Build history of the part. All positions in model axes, mm. Face numbers are marked on the shaded views. A direction names the side the tool comes from. Give positions to 0.01 mm unless a question says otherwise; leave off trailing zeros. Order: outer loops, then holes, each group sorted by start corner. A loop starts at its lowest first (then second) coordinate and runs counter-clockwise, first axis right, second up. Notation, with made-up numbers: M 54.5,51 L 77.5,51 A10 ccw 77.5,56 Z; hole C 29.25,-19 d8. An arc over 180 degrees is marked long. One line per item, written item: value.
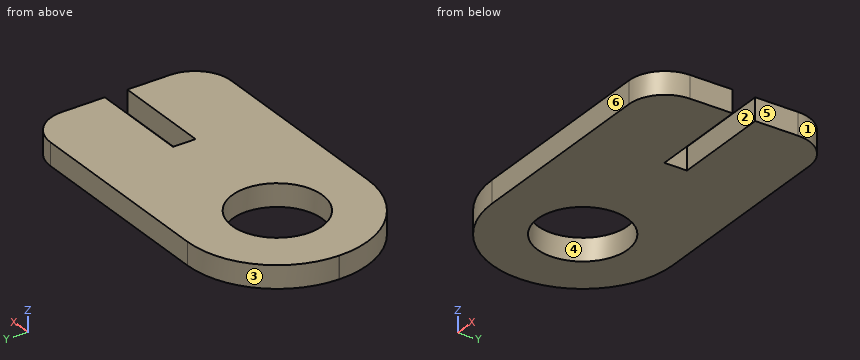
from build123d import *

# Parameters (mm, degrees)
SKETCH1_R           = 3.175
BOSS_EXTRUDE1_DEPTH = 1.5875


with BuildPart() as part:
    # Sketch1 → Boss-Extrude1 (new body)
    with BuildSketch(Plane.XY):
        with BuildLine():
            Line((-0.0254, 6.35), (13.97, 6.35))
            ThreePointArc((13.97, 6.35), (15.766051224, 5.606051224), (16.51, 3.81))
            Line((16.51, 3.81), (16.51, 0.79375))
            Line((16.51, 0.79375), (9.525, 0.79375))
            Line((9.525, 0.79375), (9.525, -0.79375))
            Line((9.525, -0.79375), (16.51, -0.79375))
            Line((16.51, -0.79375), (16.51, -3.81))
            ThreePointArc((16.51, -3.81), (15.766051224, -5.606051224), (13.97, -6.35))
            Line((13.97, -6.35), (-0.0254, -6.35))
            ThreePointArc((-0.0254, -6.35), (-4.497567548, -4.497567548), (-6.35, -0.0254))
            Line((-6.35, -0.0254), (-6.35, 0.0254))
            ThreePointArc((-6.35, 0.0254), (-4.497567548, 4.497567548), (-0.0254, 6.35))
        make_face()
        Circle(SKETCH1_R, mode=Mode.SUBTRACT)
    extrude(amount=BOSS_EXTRUDE1_DEPTH)


solid = part.part
1) Saw through at C-C, the plane x = 2.5. Write the cut outline in (y, z).
Check values:
outline: M -6.35,0 L -1.96,0 L -1.96,1.59 L -6.35,1.59 Z; M 1.96,0 L 6.35,0 L 6.35,1.59 L 1.96,1.59 Z
2) Saw through at A-A, the plane x = 11. Write the cut outline in (y, z), then the cut area to 3 significant figures.
Check values:
outline: M -6.35,0 L -0.79,0 L -0.79,1.59 L -6.35,1.59 Z; M 0.79,0 L 6.35,0 L 6.35,1.59 L 0.79,1.59 Z
area: 17.6 mm^2
3) Mould opens along X. For the marked faces 3, 4, 5 and 6 say: released by +X, released by -X, zero draft, split by the parting line, or undercut.
Check values:
face 3: released by -X
face 4: undercut
face 5: released by +X
face 6: zero draft
4) Tool access for the marked faces 1 and 2: list every direction of +Z, -Z, +X, -X, +Y, -Y with a clear straight run to the whole face (end or side of a thin tool).
Check values:
face 1: +Z, -Z, +X, +Y
face 2: +Z, -Z, +X
5) Saw through at B-B, the plane z = 1.05. Write the cut outline in (x, y) (3 decimals), then the cut area to 3 significant figures.
Check values:
outline: M -6.35,-0.025 A6.325 ccw -0.025,-6.35 L 13.97,-6.35 A2.54 ccw 16.51,-3.81 L 16.51,-0.794 L 9.525,-0.794 L 9.525,0.794 L 16.51,0.794 L 16.51,3.81 A2.54 ccw 13.97,6.35 L -0.025,6.35 A6.325 ccw -6.35,0.025 Z; hole C 0,0 d6.35
area: 228 mm^2
6) Drill centre lines: probe 1 along Y at (x, z) = (0, 0.5) (3 decimals); probe 2 along Y at (x, z) = (13.5, 0.6); probe 3 along X at (y, z) = (-1.25, 0.55). Where is each one in solid material? Low to high. Write a range as from..to.
Check values:
probe 1: -6.35..-3.175, 3.175..6.35
probe 2: -6.35..-0.79, 0.79..6.35
probe 3: -6.23..-2.92, 2.92..16.51
7) Saw through at D-D, the plane y = 5. Write the cut outline in (x, z), then the cut area to 3 significant figures.
Check values:
outline: M -3.93,0 L 16.21,0 L 16.21,1.59 L -3.93,1.59 Z
area: 32.0 mm^2
